CAD build for the part. Positions are in the model's coordinates, mm. A direction names the side the tool comes from. Give positions to 0.01 mm unless a question says otherwise; leave off trailing zeros. Order: outer loops, then holes, each group sorted by start corner. A loop starts at its lowest first (then second) coordinate and runs counter-clockwise, first axis right, second up. Notation, with made-up numbers: M 25.25,35.5 L 43.25,35.5 A28 ccw 43.25,61.5 Z; hole C 64.25,-26 d11. An arc over 180 degrees is marked long. Put each result on its own line as item: value. Start each with the question number.
1) Two-plate mould, pull along Y, no slides. Class faces 1 (the face through (253, -1, 0)), 2 (the face through (54.42, -17.58, 24.97)): released by +Y, released by -Y, zero draft, split by the parting line, or undercut.
2) Cut at B-B (z = 0). Write the cut outline in (x, y).
3) Pin check, flat tips, straight feed: pin 1 (5 mm diameter, centred on x = 115.5, y = -25.5, fed in from +Z); pin 2 (6 mm diameter, centred on x = 155, y = -17.5, fed in from +Z); pin 3 (7 mm diameter, centred on x = -100, y = -13.53, fed in from +Z); pin 4 (19 mm diameter, centred on x = 50, y = -13.53, fed in from -Z). Stop position of each tip, or through.
4) Cut at A-A (x = 50). Write the cut outline in (y, z).
5) Drill centre lines: line 1 (Z direction, x = -217.5, y = 1); line 2 (X direction, y = 6, z = -20.5); line 3 (Z direction, x = 44, y = -10.5). Where is each one in solid material? Low to high. Write a range as [from, to].
6) Cut at C-C (y = 24.5). Write the cut outline in (x, z).
7) Cut at D-D (x = 151.5). Write the cut outline in (y, z).
8) Tool access for faces 3 (the face through (3.5, -24.99, 0.72)), 4 (the face through (54.42, -17.58, -24.97)): list every direction of +Z, -Z, +X, -X, +Y, -Y with a clear straight run to the whole face (end or side of a thin tool).
```python
from build123d import *
from build123d.topology import SkipClean

# Parameters (mm, degrees)
RESSALTO_EXTRUS_O1_DEPTH          = 250
CORTE_EXTRUS_O2_REACH             = 256.063
ESBO_O4_R                         = 6
CORTE_EXTRUS_O2_DIRECTION_2_REACH = 256.063
RESSALTO_EXTRUS_O2_START          = 3
ESBO_O5_R                         = 32
RESSALTO_EXTRUS_O2_DEPTH          = 3
ESBO_O6_R                         = 32
RESSALTO_EXTRUS_O3_DEPTH          = 3


with BuildPart() as part:
    # Esboço1 → Ressalto-extrusão1 (new, symmetric)
    with BuildSketch(Plane(origin=(0, 0, 0), x_dir=(0, 0, -1), z_dir=(1, 0, 0))):
        with BuildLine():
            Line((22.115498803, 11.657817664), (27.241951671, 16.789165231))
            ThreePointArc((27.241951671, 16.789165231), (0.001842805, -31.999999947), (-27.243885188, 16.786027518))
            Line((-27.243885188, 16.786027518), (-22.115498803, 11.657817664))
            ThreePointArc((-22.115498803, 11.657817664), (0, -25), (22.115498803, 11.657817664))
        make_face()
    extrude(amount=RESSALTO_EXTRUS_O1_DEPTH, both=True)

    # Esboço4 → Corte-extrusão2 (cut, up to next)
    with BuildSketch(Plane.XY, mode=Mode.PRIVATE) as corte_extrus_o2_sk1:
        with Locations(Location((50, -13.525079078, 0), (0, 0, 180))):
            Circle(ESBO_O4_R)
    corte_extrus_o2_tool1 = extrude(corte_extrus_o2_sk1.sketch, amount=-CORTE_EXTRUS_O2_REACH, mode=Mode.PRIVATE) & part.part
    # Esboço4 → Corte-extrusão2 (cut, up to next)
    with BuildSketch(Plane.XY, mode=Mode.PRIVATE) as corte_extrus_o2_sk2:
        with Locations(Location((-100, -13.525079078, 0), (0, 0, 180))):
            Circle(ESBO_O4_R)
    corte_extrus_o2_tool2 = extrude(corte_extrus_o2_sk2.sketch, amount=-CORTE_EXTRUS_O2_REACH, mode=Mode.PRIVATE) & part.part
    add(corte_extrus_o2_tool1.solids().sort_by_distance((50, -13.525079, 0))[0], mode=Mode.SUBTRACT)
    add(corte_extrus_o2_tool2.solids().sort_by_distance((-100, -13.525079, 0))[0], mode=Mode.SUBTRACT)

    # Esboço4 → Corte-extrusão2 direction 2 (cut, up to next)
    with BuildSketch(Plane.XY, mode=Mode.PRIVATE) as corte_extrus_o2_direction_2_sk1:
        with Locations(Location((50, -13.525079078, 0), (0, 0, 180))):
            Circle(ESBO_O4_R)
    corte_extrus_o2_direction_2_tool1 = extrude(corte_extrus_o2_direction_2_sk1.sketch, amount=CORTE_EXTRUS_O2_DIRECTION_2_REACH, mode=Mode.PRIVATE) & part.part
    # Esboço4 → Corte-extrusão2 direction 2 (cut, up to next)
    with BuildSketch(Plane.XY, mode=Mode.PRIVATE) as corte_extrus_o2_direction_2_sk2:
        with Locations(Location((-100, -13.525079078, 0), (0, 0, 180))):
            Circle(ESBO_O4_R)
    corte_extrus_o2_direction_2_tool2 = extrude(corte_extrus_o2_direction_2_sk2.sketch, amount=CORTE_EXTRUS_O2_DIRECTION_2_REACH, mode=Mode.PRIVATE) & part.part
    add(corte_extrus_o2_direction_2_tool1.solids().sort_by_distance((50, -13.525079, 0))[0], mode=Mode.SUBTRACT)
    add(corte_extrus_o2_direction_2_tool2.solids().sort_by_distance((-100, -13.525079, 0))[0], mode=Mode.SUBTRACT)

    # Esboço5 → Ressalto-extrusão2 (add)
    with SkipClean():  # the faces are left unmerged after this step: merging them gives an invalid solid
        with BuildSketch(Plane(origin=(250, 0, 0), x_dir=(0, 0, -1), z_dir=(1, 0, 0)).offset(RESSALTO_EXTRUS_O2_START)):
            with Locations(Location((0, 0, 0), (0, 0, 148.36114649))):
                Circle(ESBO_O5_R)
        extrude(amount=-RESSALTO_EXTRUS_O2_DEPTH)

    # Esboço6 → Ressalto-extrusão3 (add)
    with SkipClean():  # the faces are left unmerged after this step: merging them gives an invalid solid
        with BuildSketch(Plane.ZY.offset(250)):
            Circle(ESBO_O6_R)
        extrude(amount=RESSALTO_EXTRUS_O3_DEPTH)


solid = part.part
```
Solution:
1. face 1: zero draft
1. face 2: undercut
2. outline: M -253,-32 L 253,-32 L 253,32 L 250,32 L 250,-25 L -250,-25 L -250,32 L -253,32 Z
3. pin 1: z = 22.25
3. pin 2: z = 28.53
3. pin 3: through
3. pin 4: z = -31.75
4. outline: M -19.53,-25.35 L -19.53,-15.61 A25 cw -19.53,15.61 L -19.53,25.35 A32 ccw Z; M -7.53,-31.1 A32 ccw 16.79,-27.24 L 11.66,-22.12 A25 cw -7.53,-23.84 Z; M -7.53,23.84 A25 cw 11.66,22.12 L 16.79,27.24 A32 ccw -7.53,31.1 Z
5. line 1: [-31.98, -24.98], [24.98, 31.98]
5. line 2: [-253, -250], [250, 253]
5. line 3: [-30.23, -22.69], [22.69, 30.23]
6. outline: M -253,-20.59 L -250,-20.59 L -250,20.59 L -253,20.59 Z; M 250,-20.59 L 253,-20.59 L 253,20.59 L 250,20.59 Z
7. outline: M 11.66,-22.12 A25 cw long 11.66,22.12 L 16.79,27.24 A32 ccw long 16.79,-27.24 Z
8. face 3: none
8. face 4: +Z, -Z
